Design review of the part built by this model. Coordinates are the model's own, in mm. Give positions to 0.01 mm unless a question says otherwise; leave off trailing zeros. Order: outer loops, then holes, each group sorted by start corner. A loop starts at its lowest first (then second) coordinate and runs counter-clockwise, first axis right, second up. Notation, with made-up numbers: M 4,4.5 L 22,4.5 A18 ccw 22,20.5 Z; hole C 54.25,-36.5 d5. An arc over 180 degrees is marked long. Put each result on its own line as item: value. Start each with the question number.
Autodesk Inventor part; units mm, degrees
ref_plane "YZ Plane" through (0, 0, 0) normal (1, 0, 0) x (0, 1, 0)
ref_plane "XZ Plane" through (0, 0, 0) normal (0, 1, 0) x (-1, 0, 0)
ref_plane "XY Plane" through (0, 0, 0) normal (0, 0, 1) x (1, 0, 0)
sketch "スケッチ1" plane through (0, 0, 0) normal (0, 1, 0) x (-1, 0, 0)
  line L0 (5.0263, 6.4044) -> (-44.9737, 6.4044)
  line L1 (-44.9737, 6.4044) -> (-44.9737, -43.5956)
  line L2 (-44.9737, -43.5956) -> (5.0263, -43.5956)
  line L3 (5.0263, -43.5956) -> (5.0263, 6.4044)
  point P0 (0, 0)
  dimension "d0" = 50
  dimension "d1" = 50
extrude "押し出し1" add sketch "スケッチ1" along normal blind 2
sketch "スケッチ2" plane through (0, 2, 0) normal (0, 1, 0) x (1, 0, 0)
  circle A0 centre (19.9737, 1.0956) radius 1.5
  line L0 (-5.0263, -6.4044) -> (44.9737, -6.4044)
  line L1 (-5.0263, 43.5956) -> (-5.0263, -6.4044)
  circle A1 centre (9.9737, 1.0956) radius 1.5
  circle A2 centre (29.9737, 1.0956) radius 1.5
  circle A3 centre (9.9737, 18.5956) radius 1.5
  circle A4 centre (19.9737, 18.5956) radius 1.5
  circle A5 centre (29.9737, 18.5956) radius 1.5
  point P0 (0, 0)
  dimension "d4" = 3
  dimension "d5" = 7.5
  dimension "d6" = 25
  dimension "d7" = 3
  dimension "d8" = 3
  dimension "d9" = 10
  dimension "d10" = 10
  dimension "d11" = 3
  dimension "d12" = 17.5
  dimension "d13" = 3
  dimension "d14" = 3
  dimension "d15" = 10
  dimension "d16" = 10
  dimension "d17" = 17.5
hole "穴1" at (9.9737, 2, -1.0956) at (19.9737, 2, -1.0956) at (29.9737, 2, -1.0956) at (9.9737, 2, -18.5956) at (19.9737, 2, -18.5956) at (29.9737, 2, -18.5956) direction (0, -1, 0) diameter 3 depth 2
equation "\"BendRadius\" = Thickness"
equation "\"BendReliefWidth\" = Thickness"
equation "\"BendReliefDepth\" = 0.5 * Thickness"
equation "\"CornerReliefSize\" = 4 * Thickness"
equation "\"MinimumRemnant\" = 2 * Thickness"
equation "\"TransitionRadius\" = BendRadius"
equation "\"JacobiRadiusSize\" = BendRadius"
equation "\"GapSize\" = Thickness"
properties part number "nhk20" material "アルミニウム 6061"
1. Consider section A-A on y = 0.9. Give the boundary of the cut face in (x, z).
2. Insertion check: pin 1 (1.5 mm diameter, centred on x = 1.5, z = -27, fed in from -Y); pin 2 (2.5 mm diameter, centred on x = 9.97, z = -1.1, fed in from -Y). Each pin has a flat end and moves straight along its axis. Give the tip position at first contact, or say it passes through.
3. To check wall thickness, follow probe 1 along Z at (x, y) = (20, 1.35); probe 2 along Z at (x, y) = (29.5, 0.5); probe 3 along X at (y, z) = (1.35, 0). State the ranges of each line that lie inside material, in increasing order.
4. The part is to be moulded in two halves that separate along Z. For faces 1 (the cylindrical face through (19.523, 0.986, -17.165)), 2 (the flat face through (20, 0, -24)), 3 (the flat face through (20, 1, -43.596)), say which applies: +Z half, -Z half, draft (parallel to the pull), parting line (faces both ways), or undercut.
Returned:
1. outline: M -5.03,-43.6 L 44.97,-43.6 L 44.97,6.4 L -5.03,6.4 Z; hole C 9.97,-18.6 d3; hole C 9.97,-1.1 d3; hole C 19.97,-18.6 d3; hole C 19.97,-1.1 d3; hole C 29.97,-18.6 d3; hole C 29.97,-1.1 d3
2. pin 1: stops at y = 0
2. pin 2: passes through
3. probe 1: z = -43.6 to -20.1, -17.1 to -2.6, 0.4 to 6.4
3. probe 2: z = -43.6 to -20.02, -17.17 to -2.52, 0.33 to 6.4
3. probe 3: x = -5.03 to 8.95, 11 to 18.95, 21 to 28.95, 31 to 44.97
4. face 1: undercut
4. face 2: draft
4. face 3: -Z half
